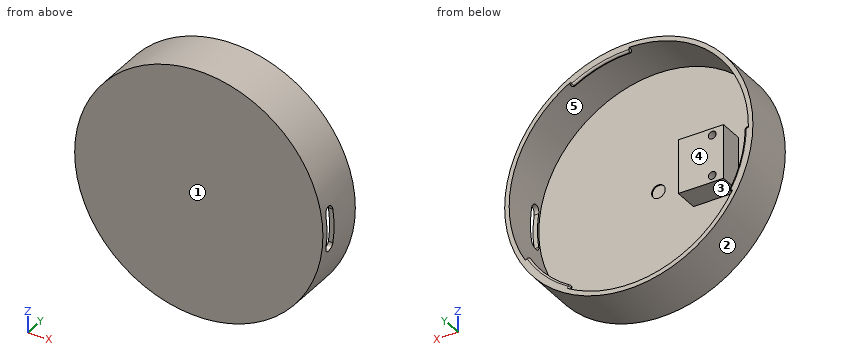
Autodesk Inventor part; units mm, degrees
ref_plane "YZ Plane" through (0, 0, 0) normal (1, 0, 0) x (0, 1, 0)
ref_plane "XZ Plane" through (0, 0, 0) normal (0, 1, 0) x (-1, 0, 0)
ref_plane "XY Plane" through (0, 0, 0) normal (0, 0, 1) x (1, 0, 0)
sketch "Sketch1" plane through (0, 0, 0) normal (0, 1, 0) x (-1, 0, 0)
  circle A0 centre (0, 0) radius 69.85
  dimension "d0" = 139.7
extrude "Extrusion1" add sketch "Sketch1" along normal blind 29.21
sketch "Sketch3" plane through (0, 29.21, 0) normal (0, 1, 0) x (1, 0, 0)
  circle A0 centre (0, 0) radius 67.31
  dimension "d5" = 134.62
extrude "Extrusion2" cut sketch "Sketch3" against normal blind 26.67
sketch "Sketch6" plane through (0, 0, 0) normal (1, 0, 0) x (0, 1, 0)
  line L0 (29.21, 67.31) -> (2.54, 67.31)
  line L1 (29.21, 67.31) -> (26.924, 67.31)
  line L2 (26.924, 67.31) -> (26.924, 65.024)
  line L3 (26.924, 65.024) -> (29.21, 65.024)
  line L4 (29.21, 65.024) -> (29.21, 67.31)
  line L5 (-5.842, 0) -> (35.052, 0)
  line L6 (29.21, -69.85) -> (29.21, 69.85)
  point P0 (0, 0)
  dimension "d21" = 2.286
  dimension "d22" = 2.286
  dimension "d36" = 0
revolve "Revolution1" add sketch "Sketch6" angle 30 about axis through (0, -10, 0) along (0, 1, 0)
fillet "Fillet2" radius 1.143 2 edges at (16.8294, 26.924, 62.8084) (16.8294, 29.21, 62.8084)
fillet "Fillet3" radius 1.143 3 edges at (32.6793, 27.2586, 56.6022) (33.3691, 29.21, 57.797) (33.3691, 26.924, 57.797)
pattern_circular "Circular Pattern1" count 3 over 360 about axis through (0, 0, 0) along (0, 1, 0) of "Revolution1", "Fillet2", "Fillet3"
sketch "Sketch9" plane through (0, 0, 0) normal (1, 0, 0) x (0, 1, 0)
  circle A0 centre (6.8717, 0) radius 3.175 construction
  line L0 (6.8717, 0) -> (6.8717, -12.7) construction
  line L1 (6.8717, 0) -> (6.8717, 12.7) construction
  line L2 (6.8717, -12.7) -> (6.8717, -12.7)
  line L3 (3.6967, -9.525) -> (3.6967, 9.525)
  line L4 (6.8717, 12.7) -> (6.8717, 12.7)
  line L5 (10.0467, 9.525) -> (10.0467, -9.525)
  arc A1 (6.8717, -12.7) -> (10.0467, -9.525) centre (6.8717, -9.525) ccw
  arc A2 (3.6967, -9.525) -> (6.8717, -12.7) centre (6.8717, -9.525) ccw
  arc A3 (6.8717, 12.7) -> (3.6967, 9.525) centre (6.8717, 9.525) ccw
  arc A4 (10.0467, 9.525) -> (6.8717, 12.7) centre (6.8717, 9.525) ccw
  point P0 (0, 0)
  dimension "d37" = 6.35
  dimension "d48" = 12.7
  dimension "d49" = 12.7
  dimension "d50" = 3.175
extrude "Extrusion9" cut sketch "Sketch9" along normal through all
sketch "Sketch15" plane through (0, 2.54, 0) normal (0, 1, 0) x (1, 0, 0)
  line L0 (-19.7435, -6.1595) -> (-19.7435, 6.1595)
  line L1 (-31.8085, -6.1595) -> (-19.7435, -6.1595)
  line L2 (-31.8085, 6.1595) -> (-19.7435, 6.1595)
  line L3 (-47.8867, -3.627) -> (-47.8867, 3.627)
  point P0 (0, 0)
sketch "Sketch16" plane through (0, 2.54, 0) normal (0, 1, 0) x (1, 0, 0)
  line L0 (-19.7435, -6.1595) -> (-19.7435, 6.1595) construction
  line L1 (-31.8085, 6.1595) -> (-19.7435, 6.1595) construction
  line L2 (-31.8085, -6.1595) -> (-19.7435, -6.1595) construction
  line L3 (-47.8867, -3.627) -> (-47.8867, 3.627) construction
  line L4 (-19.7435, 0) -> (-19.7435, 15.24)
  line L5 (-19.7435, 15.24) -> (-45.1435, 15.24)
  line L6 (-19.7435, 0) -> (-19.7435, -15.24)
  line L7 (-19.7435, -15.24) -> (-45.1435, -15.24)
  line L8 (-45.1435, -15.24) -> (-45.1435, 15.24)
  point P0 (0, 0)
  dimension "d53" = 15.24
  dimension "d54" = 25.4
  dimension "d55" = 15.24
  dimension "d56" = 25.4
extrude "Extrusion10" add sketch "Sketch16" along normal blind 13.589
sketch "Sketch17" plane through (0, 16.129, 0) normal (0, 1, 0) x (1, 0, 0)
  circle A0 centre (-38.7935, -11.43) radius 2.159
  circle A1 centre (-38.7935, 11.43) radius 2.159
  line L0 (-45.1435, -15.24) -> (-19.7435, -15.24)
  line L1 (-45.1435, 15.24) -> (-45.1435, -15.24)
  point P0 (0, 0)
  dimension "d59" = 4.318
  dimension "d60" = 4.318
  dimension "d61" = 22.86
  dimension "d62" = 3.81
  dimension "d63" = 6.35
  dimension "d64" = 6.35
extrude "Extrusion11" cut sketch "Sketch17" against normal blind 13.589
sketch "Sketch18" plane through (0, 2.54, 0) normal (0, 1, 0) x (1, 0, 0)
  circle A0 centre (0, 0) radius 3.81
  dimension "d67" = 7.62
extrude "Extrusion12" cut sketch "Sketch18" against normal blind 0.635
properties part number "bottom_basket"
Read the model definition and answer for the solid it produces. Units are mm, in the model's axes. Face numbers are marked on the shaded views. A direction names the side the tool comes from. Round coordinates to 2 decimals unless told otherwise and drop trailing zeros. Write each loop counter-clockwise with the first axis right and the second up, starting at its lowest first coordinate (ties: lowest second). Pieces come first, ordered by that corner, then holes.
1. Determine the mould class of the marked faces 1, 2 and 3 for opening direction X: pulls with the +X half, pulls with the -X half, needs draft (parallel to the pull), parting line crosses it, or undercut.
2. The part is cut by section B-B, the plane z = 42. Determine the outline of the cut face in (x, y).
3. Straight lines are drawn through the part: L1, parallel to Z at x = 2, y = 20.25; L2, parallel to X at y = 10.5, z = 11.43; L3, parallel to X at y = 9, z = -11.43. For each, find the intervals that lie inside material, in ascending order.
4. Which of the six approach directions +Z, -Z, +X, -X, +Y, -Y give full straight-line access (tool end or side, diameter ignored) to the marked faces 4 and 5?
5. The part is cut by section A-A, the plane x = -25. Determine the outline of the cut face in (y, z), then the cut area to 3 significant figures.
6. Given pin 1 Ø6 at (y, z) = (17, 22.5) entering from -X; pin 2 Ø1.8 at (y, z) = (28.5, 65.5) entering from -X; pin 3 Ø7 at (y, z) = (6, 5) entering from +X; pin 4 Ø8 at (x, z) = (-51.5, -53) entering from +Y, each flat-ended and moving along its own axis, determine where each tip first touches the part or whether it passes through.
Values:
1. face 1: needs draft
1. face 2: parting line crosses it
1. face 3: undercut
2. outline: (-55.81, 0) - (55.81, 0) - (55.81, 29.21) - (52.6, 29.21) - (52.6, 2.54) - (-52.6, 2.54) - (-52.6, 29.21) - (-55.81, 29.21) - close
3. L1: z = -69.82 to -67.28, 67.28 to 69.82
3. L2: x = -68.91 to -66.33, -45.14 to -40.95, -36.63 to -19.74, 66.33 to 68.91
3. L3: x = -68.91 to -66.33, -45.14 to -40.95, -36.63 to -19.74
4. face 4: +Y
4. face 5: none
5. outline: (0, -65.22) - (29.21, -65.22) - (29.21, -62.5) - (2.54, -62.5) - (2.54, -15.24) - (16.13, -15.24) - (16.13, 15.24) - (2.54, 15.24) - (2.54, 62.5) - (29.21, 62.5) - (29.21, 65.22) - (0, 65.22) - close
5. area: 891 mm2
6. pin 1: stops at x = -67.07
6. pin 2: stops at x = -26.57
6. pin 3: stops at x = 69.81
6. pin 4: passes through
